from build123d import *

# Parameters (mm, degrees)
SKETCH1_R          = 114.5
BASE_FLANGE1_DEPTH = 4
SKETCH2_R          = 4.6
EXTRUDE1_DEPTH     = 4
SKETCH3_R          = 5.5
EXTRUDE2_DEPTH     = 4
CIRPATTERN1_COUNT  = 8


# Sheet-metal steps are written as plain solids
with BuildPart() as part:
    # Sketch1 → Base-Flange1 (new body)
    with BuildSketch(Plane.XY):
        with BuildLine():
            Line((294, 294), (294, 350))
            Line((294, 350), (254, 350))
            Line((254, 350), (254, 320))
            ThreePointArc((254, 320), (0, 200.675105316), (-254, 320))
            Line((-254, 320), (-254, 350))
            Line((-254, 350), (-294, 350))
            Line((-294, 350), (-294, 294))
            Line((-294, 294), (-350, 294))
            Line((-350, 294), (-350, 254))
            Line((-350, 254), (-320, 254))
            ThreePointArc((-320, 254), (-200.675105316, 0), (-320, -254))
            Line((-320, -254), (-350, -254))
            Line((-350, -254), (-350, -294))
            Line((-350, -294), (-294, -294))
            Line((-294, -294), (-294, -350))
            Line((-294, -350), (-254, -350))
            Line((-254, -350), (-254, -320))
            ThreePointArc((-254, -320), (0, -200.675105316), (254, -320))
            Line((254, -320), (254, -350))
            Line((254, -350), (294, -350))
            Line((294, -350), (294, -294))
            Line((294, -294), (350, -294))
            Line((350, -294), (350, -254))
            Line((350, -254), (320, -254))
            ThreePointArc((320, -254), (200.675105316, 0), (320, 254))
            Line((320, 254), (350, 254))
            Line((350, 254), (350, 294))
            Line((350, 294), (294, 294))
        make_face()
        Circle(SKETCH1_R, mode=Mode.SUBTRACT)
    extrude(amount=BASE_FLANGE1_DEPTH)

    # Sketch2 → Extrude1 (cut)
    with BuildSketch(Plane.XY.offset(4)):
        with Locations((274, 337.5)):
            Circle(SKETCH2_R)
        with Locations((274, 307.5)):
            Circle(SKETCH2_R)
        with Locations((307.5, 274)):
            Circle(SKETCH2_R)
        with Locations((337.5, 274)):
            Circle(SKETCH2_R)
        with Locations(Location((337.5, -274, 0), (0, 0, 180))):
            Circle(SKETCH2_R)
        with Locations(Location((307.5, -274, 0), (0, 0, 180))):
            Circle(SKETCH2_R)
        with Locations(Location((274, -307.5, 0), (0, 0, 180))):
            Circle(SKETCH2_R)
        with Locations(Location((274, -337.5, 0), (0, 0, 180))):
            Circle(SKETCH2_R)
        with Locations((-274, -337.5)):
            Circle(SKETCH2_R)
        with Locations((-274, -307.5)):
            Circle(SKETCH2_R)
        with Locations((-307.5, -274)):
            Circle(SKETCH2_R)
        with Locations((-337.5, -274)):
            Circle(SKETCH2_R)
        with Locations(Location((-337.5, 274, 0), (0, 0, 180))):
            Circle(SKETCH2_R)
        with Locations(Location((-307.5, 274, 0), (0, 0, 180))):
            Circle(SKETCH2_R)
        with Locations(Location((-274, 307.5, 0), (0, 0, 180))):
            Circle(SKETCH2_R)
        with Locations(Location((-274, 337.5, 0), (0, 0, 180))):
            Circle(SKETCH2_R)
    extrude(amount=-EXTRUDE1_DEPTH, mode=Mode.SUBTRACT)

    # Sketch3 → Extrude2 (cut)
    with BuildSketch(Plane.XY.offset(4)):
        with Locations((0, 126)):
            Circle(SKETCH3_R)
    extrude2 = extrude(amount=-EXTRUDE2_DEPTH, mode=Mode.SUBTRACT)

    # CirPattern1: Extrude2 ×8 about axis
    cirpattern1_axis = Axis((0, 0, 0), (0, 0, 1))
    for i in range(1, CIRPATTERN1_COUNT):
        add(extrude2.rotate(cirpattern1_axis, i * 360 / CIRPATTERN1_COUNT), mode=Mode.SUBTRACT)


solid = part.part
Check sheet for the modelled part. Datum: model origin and axes. Units: mm. Give positions to 0.01 mm unless a question says otherwise; leave off trailing zeros. Write each loop counter-clockwise with the first axis right and the second up, starting at its lowest first coordinate (ties: lowest second). Pieces come first, ordered by that corner, then holes. Notation, with made-up numbers: M -30,-15 L 18,-15 A22 ccw 18,9 Z; hole C 81,-22 d4. An arc over 180 degrees is marked long. Use one line per item in the form item = value.
(1) Section check A-A on x = -21.5. Record the boundary of the cut face in (y, z), plus the area to 3 significant figures.
Answer block:
outline = M -201.38,0 L -112.46,0 L -112.46,4 L -201.38,4 Z; M 112.46,0 L 201.38,0 L 201.38,4 L 112.46,4 Z
area = 711 mm2
(2) Section check B-B on y = 237. Record the boundary of the cut face in (x, z), plus the area to 3 significant figures.
Answer block:
outline = M -301.04,0 L -150.52,0 L -150.52,4 L -301.04,4 Z; M 150.52,0 L 301.04,0 L 301.04,4 L 150.52,4 Z
area = 1,200 mm2
(3) Depth check by flat-ended pin: P1, Ø2, axis at x = -339, z = 2, coming from the -Y side; P2, Ø1, axis at x = -52, z = 3, coming from the -Y side; P3, Ø2, axis at x = -185, z = 3, coming from the +Y side. Enter the tip coordinate at first touch or a pass-through.
Answer block:
P1 = -294
P2 = -204.88
P3 = 258.09
(4) Draft check along X on faces 1 (the cylindrical face through (200.7, -4.1, 2)), 2 (the cylindrical face through (-4.1, -200.7, 2)), 3 (the flat face through (-79, 105, 4)). Enter one of: pulls with the +X half, pulls with the -X half, needs draft (parallel to the pull), parting line crosses it, or undercut.
Answer block:
face_1 = pulls with the +X half
face_2 = undercut
face_3 = needs draft
(5) Section check D-D on x = 185.5. Record the boundary of the cut face in (y, z), plus the area to 3 significant figures.
Answer block:
outline = M -257.75,0 L 257.75,0 L 257.75,4 L -257.75,4 Z
area = 2,060 mm2
(6) Section check C-C on z = 0.85. State how many separate pieces and enclosed holes the cut face has, plus the area to 3 significant figures.
Answer block:
separate_pieces = 1
enclosed_holes = 25
area = 205,000 mm2
(7) Material ranges on line 1 along Y through (x, z) = (-337.5, 1.05); line 2 along X through (y, z) = (321, 2.9), recorded low to high.
Answer block:
line_1 = -294 to -278.6, -269.4 to -254, 254 to 269.4, 278.6 to 294
line_2 = -294 to -254, 254 to 294
